Source: CAD feature listing. Evaluate the final solid. Frame: model axes, mm. Give positions to 0.01 mm unless a question says otherwise; leave off trailing zeros.
from build123d import *

# Parameters (mm, degrees)
CROQUIS1_R              = 22.5
CROQUIS1_R_2            = 3.5
CROQUIS1_W              = 1
CROQUIS1_H              = 7
CROQUIS1_W_2            = 7
CROQUIS1_H_2            = 1
SALIENTE_EXTRUIR1_DEPTH = 3


with BuildPart() as part:
    # Croquis1 → Saliente-Extruir1 (new body)
    with BuildSketch(Plane(origin=(0, 0, 0), x_dir=(1, 0, 0), z_dir=(0, 1, 0))):
        with Locations(Location((0, 0, 0), (0, 0, 270))):
            Circle(CROQUIS1_R)
        with Locations(Location((0, 0, 0), (0, 0, 270))):
            Circle(CROQUIS1_R_2, mode=Mode.SUBTRACT)
        with Locations((0, 18)):
            Rectangle(CROQUIS1_W, CROQUIS1_H, mode=Mode.SUBTRACT)
        Polygon((2.869496828, 21.313516555), (3.857185169, 21.15708209), (2.762143913, 14.243263706), (1.774455573, 14.399698171), align=None, mode=Mode.SUBTRACT)
        Polygon((6.168337121, 20.602223598), (7.119393637, 20.293206603), (4.956274677, 13.635810989), (4.00521816, 13.944827983), align=None, mode=Mode.SUBTRACT)
        Polygon((9.315292482, 19.38363552), (10.206299006, 18.92964502), (7.028365508, 12.692599351), (6.137358984, 13.146589851), align=None, mode=Mode.SUBTRACT)
        Polygon((12.232874427, 17.687758005), (13.041891421, 17.099972753), (8.927394655, 11.436853792), (8.118377661, 12.024639045), align=None, mode=Mode.SUBTRACT)
        Polygon((14.849242405, 15.556349186), (15.556349186, 14.849242405), (10.606601718, 9.899494937), (9.899494937, 10.606601718), align=None, mode=Mode.SUBTRACT)
        Polygon((17.099972753, 13.041891421), (17.687758005, 12.232874427), (12.024639045, 8.118377661), (11.436853792, 8.927394655), align=None, mode=Mode.SUBTRACT)
        Polygon((18.92964502, 10.206299006), (19.38363552, 9.315292482), (13.146589851, 6.137358984), (12.692599351, 7.028365508), align=None, mode=Mode.SUBTRACT)
        Polygon((20.293206603, 7.119393637), (20.602223598, 6.168337121), (13.944827983, 4.00521816), (13.635810989, 4.956274677), align=None, mode=Mode.SUBTRACT)
        Polygon((21.15708209, 3.857185169), (21.313516555, 2.869496828), (14.399698171, 1.774455573), (14.243263706, 2.762143913), align=None, mode=Mode.SUBTRACT)
        with Locations((18, 0)):
            Rectangle(CROQUIS1_W_2, CROQUIS1_H_2, mode=Mode.SUBTRACT)
        Polygon((21.313516555, -2.869496828), (21.15708209, -3.857185169), (14.243263706, -2.762143913), (14.399698171, -1.774455573), align=None, mode=Mode.SUBTRACT)
        Polygon((20.602223598, -6.168337121), (20.293206603, -7.119393637), (13.635810989, -4.956274677), (13.944827983, -4.00521816), align=None, mode=Mode.SUBTRACT)
        Polygon((19.38363552, -9.315292482), (18.92964502, -10.206299006), (12.692599351, -7.028365508), (13.146589851, -6.137358984), align=None, mode=Mode.SUBTRACT)
        Polygon((17.687758005, -12.232874427), (17.099972753, -13.041891421), (11.436853792, -8.927394655), (12.024639045, -8.118377661), align=None, mode=Mode.SUBTRACT)
        Polygon((15.556349186, -14.849242405), (14.849242405, -15.556349186), (9.899494937, -10.606601718), (10.606601718, -9.899494937), align=None, mode=Mode.SUBTRACT)
        Polygon((13.041891421, -17.099972753), (12.232874427, -17.687758005), (8.118377661, -12.024639045), (8.927394655, -11.436853792), align=None, mode=Mode.SUBTRACT)
        Polygon((10.206299006, -18.92964502), (9.315292482, -19.38363552), (6.137358984, -13.146589851), (7.028365508, -12.692599351), align=None, mode=Mode.SUBTRACT)
        Polygon((7.119393637, -20.293206603), (6.168337121, -20.602223598), (4.00521816, -13.944827983), (4.956274677, -13.635810989), align=None, mode=Mode.SUBTRACT)
        Polygon((3.857185169, -21.15708209), (2.869496828, -21.313516555), (1.774455573, -14.399698171), (2.762143913, -14.243263706), align=None, mode=Mode.SUBTRACT)
        with Locations((0, -18)):
            Rectangle(CROQUIS1_W, CROQUIS1_H, mode=Mode.SUBTRACT)
        Polygon((-2.869496828, -21.313516555), (-3.857185169, -21.15708209), (-2.762143913, -14.243263706), (-1.774455573, -14.399698171), align=None, mode=Mode.SUBTRACT)
        Polygon((-6.168337121, -20.602223598), (-7.119393637, -20.293206603), (-4.956274677, -13.635810989), (-4.00521816, -13.944827983), align=None, mode=Mode.SUBTRACT)
        Polygon((-9.315292482, -19.38363552), (-10.206299006, -18.92964502), (-7.028365508, -12.692599351), (-6.137358984, -13.146589851), align=None, mode=Mode.SUBTRACT)
        Polygon((-12.232874427, -17.687758005), (-13.041891421, -17.099972753), (-8.927394655, -11.436853792), (-8.118377661, -12.024639045), align=None, mode=Mode.SUBTRACT)
        Polygon((-14.849242405, -15.556349186), (-15.556349186, -14.849242405), (-10.606601718, -9.899494937), (-9.899494937, -10.606601718), align=None, mode=Mode.SUBTRACT)
        Polygon((-17.099972753, -13.041891421), (-17.687758005, -12.232874427), (-12.024639045, -8.118377661), (-11.436853792, -8.927394655), align=None, mode=Mode.SUBTRACT)
        Polygon((-18.92964502, -10.206299006), (-19.38363552, -9.315292482), (-13.146589851, -6.137358984), (-12.692599351, -7.028365508), align=None, mode=Mode.SUBTRACT)
        Polygon((-20.293206603, -7.119393637), (-20.602223598, -6.168337121), (-13.944827983, -4.00521816), (-13.635810989, -4.956274677), align=None, mode=Mode.SUBTRACT)
        Polygon((-21.15708209, -3.857185169), (-21.313516555, -2.869496828), (-14.399698171, -1.774455573), (-14.243263706, -2.762143913), align=None, mode=Mode.SUBTRACT)
        with Locations((-18, 0)):
            Rectangle(CROQUIS1_W_2, CROQUIS1_H_2, mode=Mode.SUBTRACT)
        Polygon((-21.313516555, 2.869496828), (-21.15708209, 3.857185169), (-14.243263706, 2.762143913), (-14.399698171, 1.774455573), align=None, mode=Mode.SUBTRACT)
        Polygon((-20.602223598, 6.168337121), (-20.293206603, 7.119393637), (-13.635810989, 4.956274677), (-13.944827983, 4.00521816), align=None, mode=Mode.SUBTRACT)
        Polygon((-19.38363552, 9.315292482), (-18.92964502, 10.206299006), (-12.692599351, 7.028365508), (-13.146589851, 6.137358984), align=None, mode=Mode.SUBTRACT)
        Polygon((-17.687758005, 12.232874427), (-17.099972753, 13.041891421), (-11.436853792, 8.927394655), (-12.024639045, 8.118377661), align=None, mode=Mode.SUBTRACT)
        Polygon((-15.556349186, 14.849242405), (-14.849242405, 15.556349186), (-9.899494937, 10.606601718), (-10.606601718, 9.899494937), align=None, mode=Mode.SUBTRACT)
        Polygon((-13.041891421, 17.099972753), (-12.232874427, 17.687758005), (-8.118377661, 12.024639045), (-8.927394655, 11.436853792), align=None, mode=Mode.SUBTRACT)
        Polygon((-10.206299006, 18.92964502), (-9.315292482, 19.38363552), (-6.137358984, 13.146589851), (-7.028365508, 12.692599351), align=None, mode=Mode.SUBTRACT)
        Polygon((-7.119393637, 20.293206603), (-6.168337121, 20.602223598), (-4.00521816, 13.944827983), (-4.956274677, 13.635810989), align=None, mode=Mode.SUBTRACT)
        Polygon((-3.857185169, 21.15708209), (-2.869496828, 21.313516555), (-1.774455573, 14.399698171), (-2.762143913, 14.243263706), align=None, mode=Mode.SUBTRACT)
    extrude(amount=SALIENTE_EXTRUIR1_DEPTH)


solid = part.part
1) Ray query, probe 1 along X at (y, z) = (1.25, 0); probe 2 along Z at (x, y) = (8, 1.5). Return the intervals inside material, ascending.
Checks:
probe 1: x = -22.5 to -21.5, -14.5 to -3.5, 3.5 to 14.5, 21.5 to 22.5
probe 2: z = -21.03 to -16.8, -14.6 to 14.6, 16.8 to 21.03
2) Contact query for flat-ended pins moving along their axis: P1, Ø1.5, axis at y = 2, z = -13.5, coming from the +X side; P2, Ø0.5, axis at y = 1.5, z = 0, coming from the -X side; P3, Ø1.5, axis at x = -19.5, y = 2, coming from the +Z side. Output: stop coordinate, or through.
Checks:
P1: stops at x = 18.54
P2: stops at x = -22.5
P3: stops at z = 12.44
3) Pull-direction query (X, two-part tool) for faces 1 (the flat face through (-10.956, 1.479, -14.229)), 2 (the cylindrical face through (-8.618, 1.479, 20.784)); classes: released by +X, released by -X, zero draft, split by the parting line, or undercut.
Checks:
face 1: undercut
face 2: split by the parting line
4) Cut plane A-A (y = 1.05). State how many separate pieces and enclosed holes the cut face has, and give its area (3 significant figures).
Checks:
separate pieces: 1
enclosed holes: 41
area: 1,270 mm2
